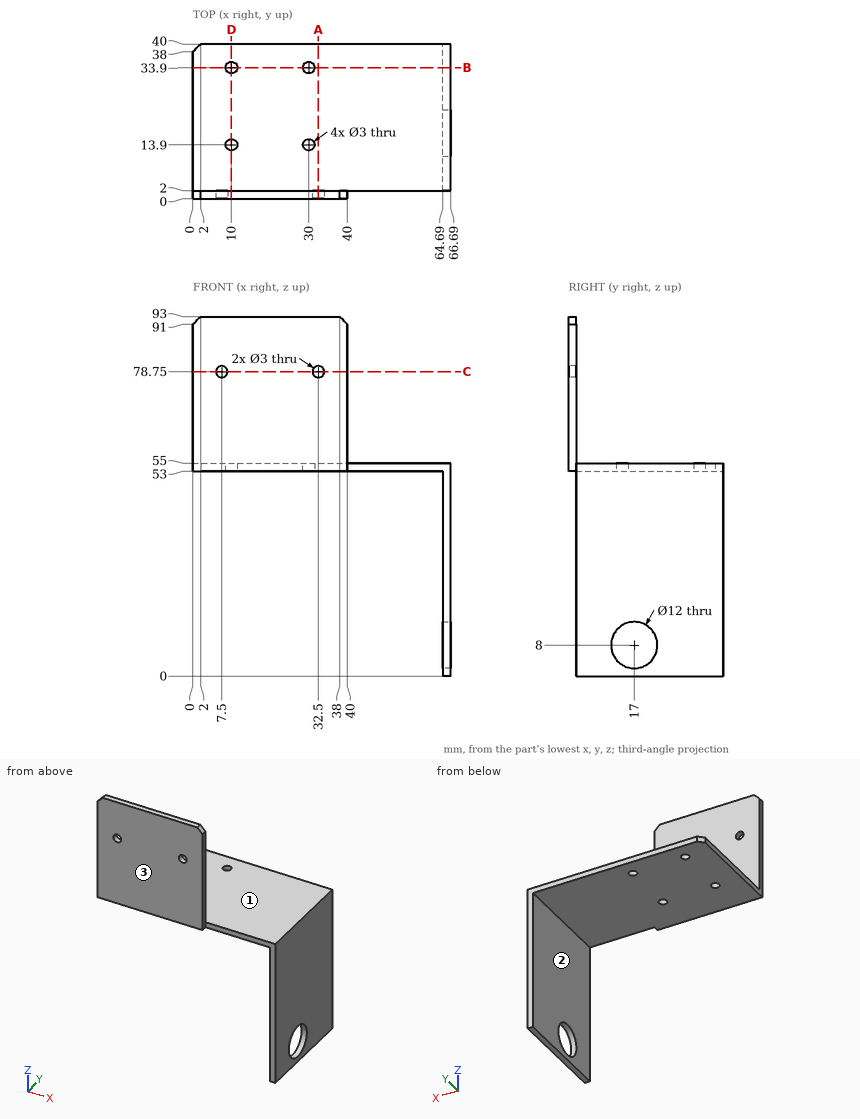
Input: dimensioned drawing with shaded views. Units: mm. Origin: part minimum x, y, z. A direction names the side the tool comes from. Round coordinates to 2 decimals unless told otherwise and drop trailing zeros. Loops run counter-clockwise (first coordinate to the right, second up) from the corner with the lowest first, then second, coordinate; pieces in that order, holes last.
1) Section query D-D on x = 10. Return the cut outline in (y, z).
Ans:
outline: (0, 53) - (12.4, 53) - (12.4, 55) - (2, 55) - (2, 93) - (0, 93) - close; (15.4, 53) - (32.4, 53) - (32.4, 55) - (15.4, 55) - close; (35.4, 53) - (40, 53) - (40, 55) - (35.4, 55) - close
2) Section query C-C on z = 78.75. Return the cut outline in (x, y), plus the area to 3 significant figures.
Ans:
outline: (0, 0) - (6, 0) - (6, 2) - (0, 2) - close; (9, 0) - (31, 0) - (31, 2) - (9, 2) - close; (34, 0) - (40, 0) - (40, 2) - (34, 2) - close
area: 68.0 mm2
3) Section query B-B on y = 33.9. Return the cut outline in (x, z), plus the area to 3 significant figures.
Ans:
outline: (0, 53) - (8.5, 53) - (8.5, 55) - (0, 55) - close; (11.5, 53) - (28.5, 53) - (28.5, 55) - (11.5, 55) - close; (31.5, 53) - (64.69, 53) - (64.69, 0) - (66.69, 0) - (66.69, 55) - (31.5, 55) - close
area: 227 mm2
4) Material intervals for line 1 (Y direction, x = 10, z = 54.1); line 2 (X direction, y = 1.05, z = 78.75); line 3 (Y direction, x = 16, z = 57), sorted ascending.
Ans:
line 1: y = 0 to 12.4, 15.4 to 32.4, 35.4 to 40
line 2: x = 0 to 6, 9 to 31, 34 to 40
line 3: y = 0 to 2
5) Pin query (flat end, axial travel): pin 1 (3.5 mm diameter, centred on x = 10, y = 33.9, fed in from +Z); pin 2 (10 mm diameter, centred on x = 31.5, z = 56, fed in from -Y); pin 3 (2 mm diameter, centred on x = 14.5, y = 25.5, fed in from -Z); pin 4 (11.5 mm diameter, centred on x = 13, z = 78, fed in from +Y). Return the tip coordinate at first contact, or that it passes through.
Ans:
pin 1: stops at z = 55
pin 2: stops at y = 0
pin 3: stops at z = 53
pin 4: stops at y = 2
6) Section query A-A on x = 32.5. Return the cut outline in (y, z), plus the area to 3 significant figures.
Ans:
outline: (0, 53) - (40, 53) - (40, 55) - (2, 55) - (2, 77.25) - (0, 77.25) - close; (0, 80.25) - (2, 80.25) - (2, 93) - (0, 93) - close
area: 150 mm2
7) Set-up query: the marked faces 1, 2 and 3. Return all of +Z, -Z, +X, -X, +Y, -Y with unobstructed straight access to the full face (end or side cutting, diameter ignored); none if empty.
Ans:
face 1: +Z, +X, -X, +Y
face 2: -Z, -X, +Y, -Y
face 3: +Z, -Z, +X, -X, -Y
